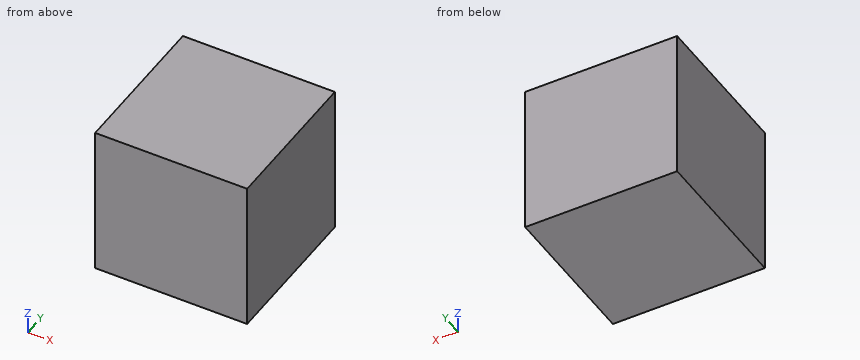
```python
from build123d import *

# Parameters (mm, degrees)
SKETCH1_W           = 50.8
SKETCH1_H           = 50.8
SKETCH1_W_2         = 38.1
SKETCH1_H_2         = 38.1
EXTRUDE_THIN1_DEPTH = 50.8
SKETCH2_W           = 38.1
SKETCH2_H           = 38.108160065
BOSS_EXTRUDE1_DEPTH = 6.35
SKETCH3_W           = 38.1
SKETCH3_H           = 38.108160065
BOSS_EXTRUDE3_DEPTH = 6.35


with BuildPart() as part:
    # Sketch1 → Extrude-Thin1 (new body)
    with BuildSketch(Plane(origin=(0, 0, 0), x_dir=(1, 0, 0), z_dir=(0, 1, 0))):
        with Locations((25.4, 25.4)):
            Rectangle(SKETCH1_W, SKETCH1_H)
        with Locations((25.4, 25.4)):
            Rectangle(SKETCH1_W_2, SKETCH1_H_2, mode=Mode.SUBTRACT)
    extrude(amount=EXTRUDE_THIN1_DEPTH)

    # Sketch2 → Boss-Extrude1 (add)
    with BuildSketch(Plane(origin=(0, 50.8, 0), x_dir=(1, 0, 0), z_dir=(0, 1, 0))):
        with Locations((25.4, 25.404080033)):
            Rectangle(SKETCH2_W, SKETCH2_H)
    extrude(amount=-BOSS_EXTRUDE1_DEPTH)

    # Sketch3 → Boss-Extrude3 (add)
    with BuildSketch(Plane.XZ):
        with Locations((25.4, -25.395919968)):
            Rectangle(SKETCH3_W, SKETCH3_H)
    extrude(amount=-BOSS_EXTRUDE3_DEPTH)


solid = part.part
```
The listing builds one solid part. Answer for the finished solid, in the listing's coordinates (mm). Give positions to 0.01 mm unless a question says otherwise; leave off trailing zeros. Order: outer loops, then holes, each group sorted by start corner. A loop starts at its lowest first (then second) coordinate and runs counter-clockwise, first axis right, second up. Notation, with made-up numbers: (3, -1) -> (8, -1) arc R26 ccw to (8, 34) -> close; hole circle Ø9 at (36.25, 73.25). An arc over 180 degrees is marked (long way). Answer as a JSON object with one key per item and string values. Group by question number.
Item 1: Consider L1, parallel to Z at x = 21, y = 32; L2, parallel to X at y = 41, z = -7.5. Determine where each line is inside the solid, lowest interval first. Write a range as from..to.
Item 2: The part is cut by section B-B on z = -10. Write down the section's boundary in (x, y), and give its area (3 significant figures).
Item 3: The part is cut by section A-A on x = 12. Write down the section's boundary in (y, z), and give its area (3 significant figures).
Result set:
{
 "1": {"L1": "-50.8..-44.45, -6.35..0", "L2": "0..6.35, 44.45..50.8"},
 "2": {"outline": "(0, 0) -> (50.8, 0) -> (50.8, 50.8) -> (0, 50.8) -> close; hole (6.35, 6.35) -> (44.45, 6.35) -> (44.45, 44.45) -> (6.35, 44.45) -> close", "area": "1,130 mm²"},
 "3": {"outline": "(0, -50.8) -> (50.8, -50.8) -> (50.8, 0) -> (0, 0) -> close; hole (6.35, -44.45) -> (44.45, -44.45) -> (44.45, -6.35) -> (6.35, -6.35) -> close", "area": "1,130 mm²"}
}
